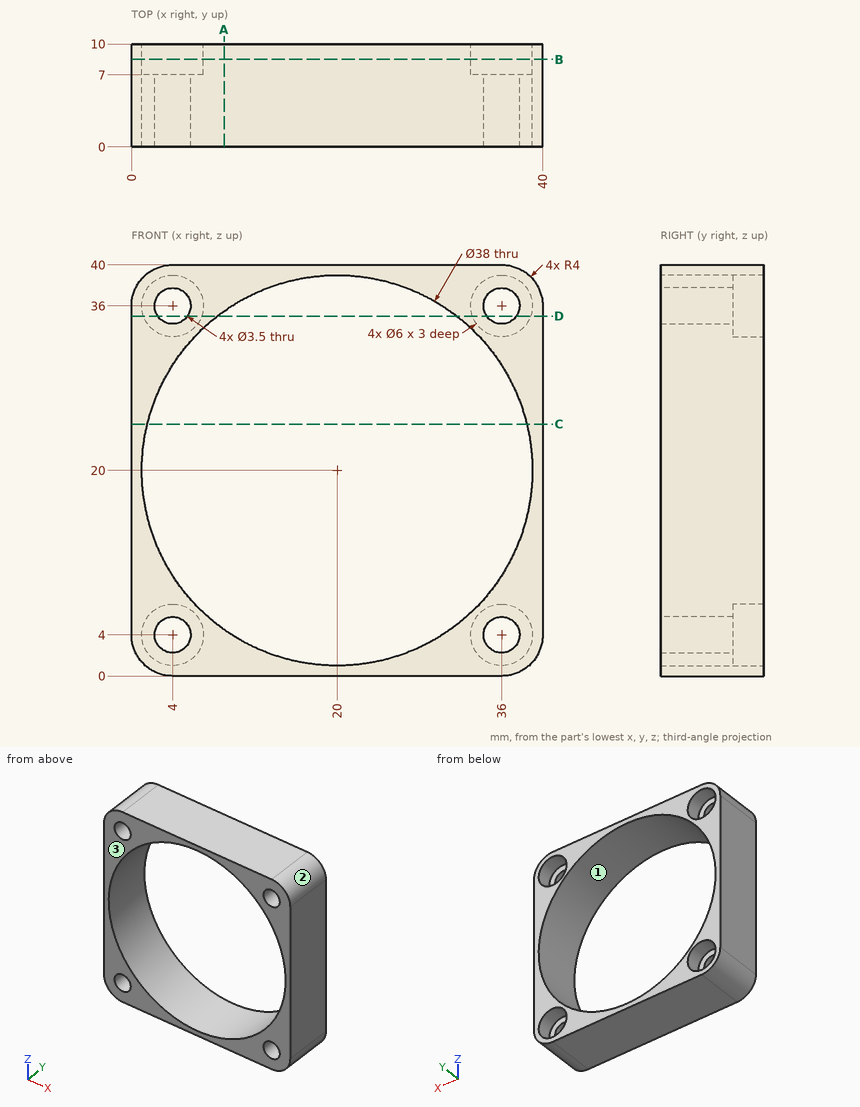
Could you check a few things on this drawing? It's one solid part, dimensions in mm from its lowest x, y, z. Round coordinates to 2 decimals unless told otherwise and drop trailing zeros. Write each loop counter-clockwise with the first axis right and the second up, starting at its lowest first coordinate (ties: lowest second). Pieces come first, ordered by that corner, then holes.
Q1. If we section it at B-B on y = 8.5: Write out the boundary of the cut face in (x, z).
Q2. Will this pin go through, and if not, where does the flat tip stop? P1, Ø3, axis at x = 37, z = 5, coming from the +Y side.
Q3. If we section it at C-C on z = 24.5: Write out the boundary of the cut face in (x, y), plus the area to 3 significant figures.
Q4. If we section it at A-A on x = 9: Write out the boundary of the cut face in (y, z).
Q5. Please list where these lines run through material, in increasing order: probe 1 along X at (y, z) = (2.25, 36); probe 2 along X at (y, z) = (7.85, 4); probe 3 along Z at (x, y) = (35.5, 9.5).
Q6. If we section it at D-D on z = 35: Write out the boundary of the cut face in (x, y), plus the area to 3 significant figures.
Q7. If we mould it in two halves opening along X, with no side actions, what happens to the marked faces 1, 2 and 3? For each: +X half, -X half, draft (parallel to the pull), parting line (faces both ways), or undercut.
Answer below:
1. outline: (0, 4) arc R4 ccw to (4, 0) - (36, 0) arc R4 ccw to (40, 4) - (40, 36) arc R4 ccw to (36, 40) - (4, 40) arc R4 ccw to (0, 36) - close; hole circle Ø6 at (4, 4); hole circle Ø38 at (20, 20); hole circle Ø6 at (4, 36); hole circle Ø6 at (36, 4); hole circle Ø6 at (36, 36)
2. P1: stops at y = 7
3. outline: (0, 0) - (1.54, 0) - (1.54, 10) - (0, 10) - close; (38.46, 0) - (40, 0) - (40, 10) - (38.46, 10) - close
3. area: 30.8 mm2
4. outline: (0, 0) - (10, 0) - (10, 4.51) - (0, 4.51) - close; (0, 35.49) - (10, 35.49) - (10, 40) - (0, 40) - close
5. probe 1: x = 0 to 2.25, 5.75 to 9.75, 30.25 to 34.25, 37.75 to 40
5. probe 2: x = 0 to 1, 7 to 9.75, 30.25 to 33, 39 to 40
5. probe 3: z = 0 to 1.04, 6.96 to 9.01, 30.99 to 33.04, 38.96 to 40
6. outline: (0, 0) - (2.56, 0) - (2.56, 7) - (1.17, 7) - (1.17, 10) - (0, 10) - close; (5.44, 0) - (8.34, 0) - (8.34, 10) - (6.83, 10) - (6.83, 7) - (5.44, 7) - close; (31.66, 0) - (34.56, 0) - (34.56, 7) - (33.17, 7) - (33.17, 10) - (31.66, 10) - close; (37.44, 0) - (40, 0) - (40, 10) - (38.83, 10) - (38.83, 7) - (37.44, 7) - close
6. area: 92.6 mm2
7. face 1: undercut
7. face 2: +X half
7. face 3: draft
